Design review of the part built by this model. Coordinates are the model's own, in mm. Give positions to 0.01 mm unless a question says otherwise; leave off trailing zeros. Loops run counter-clockwise (first coordinate to the right, second up) from the corner with the lowest first, then second, coordinate; pieces in that order, holes last. Notation, with made-up numbers: (-19, 71) -> (22, 71) arc R25 cw to (22, 109) -> close; hole circle Ø5 at (51, 85). An arc over 180 degrees is marked (long way). Use CSV: the item, a comma, the result in double quotes. Start each with the question number.
Item 1: We need section B-B (z = 35). State the section outline as (x, y) points.
Item 2: Wall thickness on line 1 along Z through (x, y) = (0.65, 113); line 2 along Z through (x, y) = (0.2, 113.5); line 3 along Y through (x, z) = (0.9, -74): over which ranges is each line inside the solid? List them lowest first. Write a range as from..to.
Item 3: The part is to be moulded in two halves that separate along Z. For faces 1 (the face through (0.74, 92.666, -1.684)), 2 (the face through (1.5, 105, 43)), 3 (the face through (0.74, 118.206, 169.039)), say which applies: +Z half, -Z half, draft (parallel to the pull), parting line (faces both ways), or undercut.
Item 4: We need section A-A (x = 1.25). Count the separate pieces of the cut face and the enclosed holes in it, plus the area to 3 significant figures.
from build123d import *

# Parameters (mm, degrees)
SKETCH_1_R      = 1.925
EXTRUDE_1_DEPTH = 1.5


with BuildPart() as part:
    # 草圖1 → 填料-伸長1 (new body)
    with BuildSketch(Plane(origin=(0, 0, 0), x_dir=(0, 0, -1), z_dir=(1, 0, 0))):
        with BuildLine():
            ThreePointArc((-130.897263822, 87.591071909), (-168.871615346, 100.442909595), (-208.309414447, 107.64576373))
            ThreePointArc((-208.309414447, 107.64576373), (-214.28117701, 115.199320657), (-206.405854958, 120.739850681))
            ThreePointArc((-206.405854958, 120.739850681), (-168.506781938, 118.224744692), (-130.897263822, 123.534136472))
            ThreePointArc((-130.897263822, 123.534136472), (-125.884787037, 124.325252138), (-121.053064598, 122.774366651))
            ThreePointArc((-121.053064598, 122.774366651), (-115.359208766, 120.190083617), (-109.218730551, 119.009812321))
            ThreePointArc((-109.218730551, 119.009812321), (1.650442282, 115.351316794), (112.469361248, 120.30361659))
            ThreePointArc((112.469361248, 120.30361659), (122.671923792, 111.836409472), (114.393924171, 101.479740068))
            ThreePointArc((114.393924171, 101.479740068), (0.082126176, 92.557578457), (-114.38926471, 85.993068006))
            ThreePointArc((-114.38926471, 85.993068006), (-122.70068315, 86.198910651), (-130.897263822, 87.591071909))
        make_face()
        with Locations((113.258391089, 110.873964994)):
            Circle(SKETCH_1_R, mode=Mode.SUBTRACT)
        with Locations((-207.723896624, 114.246052716)):
            Circle(SKETCH_1_R, mode=Mode.SUBTRACT)
        with Locations((-78.841316581, 102.391494034)):
            Circle(SKETCH_1_R, mode=Mode.SUBTRACT)
        with Locations((-126.72836608, 113.395152076)):
            Circle(SKETCH_1_R, mode=Mode.SUBTRACT)
        with Locations((75.716339506, 107.068132225)):
            Circle(SKETCH_1_R, mode=Mode.SUBTRACT)
    extrude(amount=EXTRUDE_1_DEPTH)


solid = part.part
Results found:
1,outline,"(0, 90.29) -> (1.5, 90.29) -> (1.5, 115.61) -> (0, 115.61) -> close"
2,line 1,"-122.48..124.84, 128.61..206.26, 209.19..214.23"
2,line 2,"-122.35..124.81, 128.65..205.95, 209.5..214.31"
2,line 3,"98.06..106.2, 107.94..117.61"
3,face 1,"-Z half"
3,face 2,"draft"
3,face 3,"undercut"
4,separate pieces,"1"
4,enclosed holes,"5"
4,area,"7,740 mm²"
